Geometry check sheet. Reference: the model listing, model coordinates, mm. Face numbers are marked on the shaded views. A direction names the side the tool comes from. Give positions to 0.01 mm unless a question says otherwise; leave off trailing zeros. Loops run counter-clockwise (first coordinate to the right, second up) from the corner with the lowest first, then second, coordinate; pieces in that order, holes last.
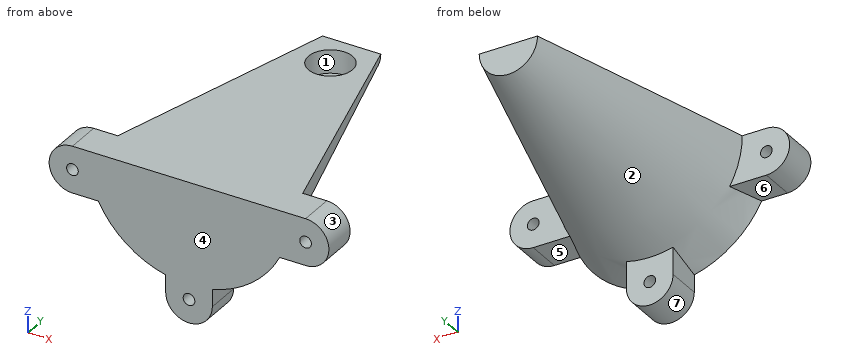
```python
from build123d import *

# Parameters (mm, degrees)
SKETCH3_R           = 1.27
BOSS_EXTRUDE1_DEPTH = 7.62
SKETCH4_R           = 4.8006
CUT_EXTRUDE1_DEPTH  = 5.08


with BuildPart() as part:
    # Sketch1 → Loft1 section 0
    with BuildSketch(Plane(origin=(0, 0, 0), x_dir=(1, 0, 0), z_dir=(0, 1, 0))):
        with BuildLine():
            Line((-22.225, 0), (22.225, 0))
            ThreePointArc((22.225, 0), (0, 22.225), (-22.225, 0))
        make_face()
    # Sketch2 → Loft1 section 1
    with BuildSketch(Plane(origin=(0, 58.42, 0), x_dir=(1, 0, 0), z_dir=(0, 1, 0))):
        with BuildLine():
            Line((-6.35, 0), (6.35, 0))
            ThreePointArc((6.35, 0), (0, 6.35), (-6.35, 0))
        make_face()
    loft()

    # Sketch3 → Boss-Extrude1 (add)
    with BuildSketch(Plane(origin=(0, 0, 0), x_dir=(1, 0, 0), z_dir=(0, 1, 0))):
        with BuildLine():
            Line((5.08, 25.4), (5.08, 10.16))
            Line((5.08, 10.16), (25.4, 10.16))
            ThreePointArc((25.4, 10.16), (30.48, 5.08), (25.4, 0))
            Line((25.4, 0), (-25.4, 0))
            ThreePointArc((-25.4, 0), (-30.48, 5.08), (-25.4, 10.16))
            Line((-25.4, 10.16), (-5.08, 10.16))
            Line((-5.08, 10.16), (-5.08, 25.4))
            ThreePointArc((-5.08, 25.4), (0, 30.48), (5.08, 25.4))
        make_face()
        with Locations(Location((25.4, 5.08, 0), (0, 0, 90))):
            Circle(SKETCH3_R, mode=Mode.SUBTRACT)
        with Locations(Location((-25.4, 5.08, 0), (0, 0, 90))):
            Circle(SKETCH3_R, mode=Mode.SUBTRACT)
        with Locations(Location((0, 25.4, 0), (0, 0, 90))):
            Circle(SKETCH3_R, mode=Mode.SUBTRACT)
    extrude(amount=BOSS_EXTRUDE1_DEPTH)

    # Sketch4 → Cut-Extrude1 (cut)
    with BuildSketch(Plane.XY):
        with Locations((0, 50.8)):
            Circle(SKETCH4_R)
    extrude(amount=-CUT_EXTRUDE1_DEPTH, mode=Mode.SUBTRACT)


solid = part.part
```
1) Sectioned sample at C-C on y = 24.5. Enter the section's corners in (x, z).
2) Tool access check on the marked faces 5, 6 and 7. Record the directions out of +Z, -Z, +X, -X, +Y, -Y that give a thin tool (end or side, any length) a straight path to the whole face; none if there is none.
3) Depth check by flat-ended pin: P1, Ø6, axis at x = 20, y = 2.5, coming from the -Z side; P2, Ø3, axis at x = 0, z = -25.4, coming from the +Y side; P3, Ø8.5, axis at x = -20.5, y = 3, coming from the -Z side. Enter the tip coordinate at first touch or a pass-through.
4) Sectioned sample at A-A on x = 0. Enter the section's corners in (y, z), plus the area to 3 significant figures.
5) Mould release check, pull along Y, two halves, no side actions. Record for the marked faces 1, 2, 3 and 4: +Y half, -Y half, draft (parallel to the pull), parting line (faces both ways), or undercut.
6) Sectioned sample at B-B on y = 32. Enter the section's corners in (x, z), plus the area to 3 significant figures.
7) Scan lines: line 1 along X through (y, z) = (3, -5.08); line 2 along Y through (x, z) = (0, -2.6); line 3 along Z through (x, y) = (-25.4, 5.75). Record each from-to range of solid material in increasing order.
Determined:
1. outline: (-15.57, 0) arc R15.57 ccw to (15.57, 0) - close
2. face 5: -Z, +X, +Y
2. face 6: -Z, -X, +Y
2. face 7: -Z, +Y, -Y
3. P1: stops at z = -13.46
3. P2: stops at y = 7.62
3. P3: stops at z = -14.25
4. outline: (0, -30.48) - (7.62, -30.48) - (7.62, -26.67) - (0, -26.67) - close; (0, -24.13) - (7.62, -24.13) - (7.62, -20.15) - (58.42, -6.35) - (58.42, 0) - (55.6, 0) - (55.6, -5.08) - (46, -5.08) - (46, 0) - (0, 0) - close
4. area: 837 mm2
5. face 1: undercut
5. face 2: +Y half
5. face 3: draft
5. face 4: -Y half
6. outline: (-13.53, 0) arc R13.53 ccw to (13.53, 0) - close
6. area: 288 mm2
7. line 1: x = -30.48 to -26.67, -24.13 to 24.13, 26.67 to 30.48
7. line 2: y = 0 to 46, 55.6 to 58.42
7. line 3: z = -10.16 to -6.35, -3.81 to 0
